Work out the finished part from the listing and answer in its coordinate system (mm). A direction names the side the tool comes from. Coordinates: 2 decimals unless noted, no trailing zeros. Write each loop counter-clockwise with the first axis right and the second up, starting at its lowest first coordinate (ties: lowest second). Pieces come first, ordered by that corner, then holes. Notation, with made-up numbers: (65, 33.5) - (116, 33.5) arc R32 cw to (116, 64.5) - close; hole circle Ø7 at (54, -36.75). An arc over 180 degrees is marked (long way). One line per item, written item: value.
```python
from build123d import *

# Parameters (mm, degrees)
SKETCH1_R               = 15.875
BOSS_EXTRUDE1_DEPTH     = 4.318
SKETCH4_R               = 9.398
BOSS_EXTRUDE2_DEPTH     = 12.954
SKETCH5_R               = 2.921
CUT_EXTRUDE1_DEPTH      = 26.919825732
CUT_EXTRUDE1_DEPTH_BACK = 3.302
SKETCH6_R               = 1.4605
SKETCH6_R_2             = 1.73706236
CUT_EXTRUDE2_DEPTH      = 26.919825732
CUT_EXTRUDE2_DEPTH_BACK = 26.919825732
SKETCH10_R              = 1.27
CUT_EXTRUDE6_DEPTH      = 29.325840394
SKETCH12_R              = 9.398
SKETCH12_R_2            = 8.4455
CUT_EXTRUDE8_DEPTH      = 11.684
CUT_EXTRUDE9_DEPTH      = 10.16


with BuildPart() as part:
    # Sketch1 → Boss-Extrude1 (new body)
    with BuildSketch(Plane(origin=(0, 0, 0), x_dir=(1, 0, 0), z_dir=(0, 1, 0))):
        with Locations(Location((0, 0, 0), (0, 0, 270))):
            Circle(SKETCH1_R)
    extrude(amount=BOSS_EXTRUDE1_DEPTH)

    # Sketch4 → Boss-Extrude2 (add)
    with BuildSketch(Plane(origin=(0, 4.318, 0), x_dir=(1, 0, 0), z_dir=(0, 1, 0))):
        with Locations(Location((0, 0, 0), (0, 0, 270))):
            Circle(SKETCH4_R)
    extrude(amount=BOSS_EXTRUDE2_DEPTH)

    # Sketch5 → Cut-Extrude1 (cut, two sides)
    with BuildSketch(Plane(origin=(0, 4.318, 0), x_dir=(1, 0, 0), z_dir=(0, 1, 0))) as cut_extrude1_sk:
        with Locations(Location((-11.43, 0, 0), (0, 0, 40.395058429))):
            Circle(SKETCH5_R)
        with Locations(Location((11.43, 0, 0), (0, 0, 139.604941571))):
            Circle(SKETCH5_R)
    extrude(amount=CUT_EXTRUDE1_DEPTH, mode=Mode.SUBTRACT)
    extrude(cut_extrude1_sk.sketch, amount=-CUT_EXTRUDE1_DEPTH_BACK, mode=Mode.SUBTRACT)

    # Sketch6 → Cut-Extrude2 (cut, two sides)
    with BuildSketch(Plane(origin=(0, 4.318, 0), x_dir=(1, 0, 0), z_dir=(0, 1, 0))) as cut_extrude2_sk:
        with Locations(Location((-11.43, 0, 0), (0, 0, 270))):
            Circle(SKETCH6_R)
        with Locations(Location((11.43, 0, 0), (0, 0, 270))):
            Circle(SKETCH6_R_2)
    extrude(amount=CUT_EXTRUDE2_DEPTH, mode=Mode.SUBTRACT)
    extrude(cut_extrude2_sk.sketch, amount=-CUT_EXTRUDE2_DEPTH_BACK, mode=Mode.SUBTRACT)

    # Sketch10 → Cut-Extrude6 (cut, through all)
    with BuildSketch(Plane(origin=(0, 17.272, 0), x_dir=(1, 0, 0), z_dir=(0, 1, 0))):
        with Locations(Location((0, 5.08, 0), (0, 0, 270))):
            Circle(SKETCH10_R)
        with Locations(Location((0, -5.08, 0), (0, 0, 270))):
            Circle(SKETCH10_R)
        with Locations(Location((5.08, 0, 0), (0, 0, 270))):
            Circle(SKETCH10_R)
        with Locations(Location((-5.08, 0, 0), (0, 0, 270))):
            Circle(SKETCH10_R)
    extrude(amount=-CUT_EXTRUDE6_DEPTH, mode=Mode.SUBTRACT)

    # Sketch12 → Cut-Extrude8 (cut)
    with BuildSketch(Plane(origin=(0, 17.272, 0), x_dir=(1, 0, 0), z_dir=(0, 1, 0))):
        Circle(SKETCH12_R)
        with Locations(Location((0, 0, 0), (0, 0, 270))):
            Circle(SKETCH12_R_2, mode=Mode.SUBTRACT)
    extrude(amount=-CUT_EXTRUDE8_DEPTH, mode=Mode.SUBTRACT)

    # Sketch13 → Cut-Extrude9 (cut)
    with BuildSketch(Plane.XZ):
        Polygon((7.426351494, 0), (6.253175747, 2.032), (3.906824253, 2.032), (2.733648506, 0), (3.906824253, -2.032), (6.253175747, -2.032), align=None)
        Polygon((2.346351494, -5.08), (1.173175747, -3.048), (-1.173175747, -3.048), (-2.346351494, -5.08), (-1.173175747, -7.112), (1.173175747, -7.112), align=None)
        Polygon((-2.733648506, 0), (-3.906824253, 2.032), (-6.253175747, 2.032), (-7.426351494, 0), (-6.253175747, -2.032), (-3.906824253, -2.032), align=None)
        Polygon((2.346351494, 5.08), (1.173175747, 7.112), (-1.173175747, 7.112), (-2.346351494, 5.08), (-1.173175747, 3.048), (1.173175747, 3.048), align=None)
    extrude(amount=-CUT_EXTRUDE9_DEPTH, mode=Mode.SUBTRACT)


solid = part.part
```
Item 1: Given pin 1 (1.2 mm diameter, centred on x = 0.5, z = 5, fed in from -Y); pin 2 (6 mm diameter, centred on x = -12.5, y = 3, fed in from -Z); pin 3 (8 mm diameter, centred on x = 8.5, y = 12.5, fed in from -Z); pin 4 (0.7 mm diameter, centred on x = -5.5, y = 7, fed in from +Z), each flat-ended and moving along its own axis, determine where each tip first touches the part or whether it passes through.
Evaluation:
pin 1: passes through
pin 2: stops at z = -12.72
pin 3: stops at z = -7.15
pin 4: stops at z = 6.69
Item 2: Determine the mould class of faces 4 (the face through (-0.18, 4.944, 9.396)), 5 (the face through (1.75, 5.01, -6.11)), 6 (the face through (0, 17.272, 0)) for opening direction X: +X half, -X half, draft (parallel to the pull), parting line (faces both ways), or undercut.
Evaluation:
face 4: parting line
face 5: undercut
face 6: draft
Item 3: Section A-A, the plane x = 0 is taken. Give the number of separate pieces and of enclosed holes in the cut face, then the cut area to 3 significant figures.
Evaluation:
separate pieces: 3
enclosed holes: 0
area: 240 mm2
Item 4: Which of the six approach directions +Z, -Z, +X, -X, +Y, -Y give full straight-line access (tool end or side, diameter ignored) to faces 1 (the face through (-1.77, 5.01, -6.08)), 2 (the face through (2.537, 11.512, 8.056)), 3 (the face through (-12.856, 0.515, -0.317))?
Evaluation:
face 1: -Y
face 2: +Y
face 3: +Y, -Y
Item 5: Section B-B, the plane y = 3.5 is taken. Determine the outline of the cut face in (x, z) (3 decimals).
Evaluation:
outline: circle Ø31.75 at (0, 0); hole circle Ø5.842 at (-11.43, 0); hole (-7.426, 0) - (-6.253, -2.032) - (-3.907, -2.032) - (-2.734, 0) - (-3.907, 2.032) - (-6.253, 2.032) - close; hole (-2.346, -5.08) - (-1.173, -7.112) - (1.173, -7.112) - (2.346, -5.08) - (1.173, -3.048) - (-1.173, -3.048) - close; hole (-2.346, 5.08) - (-1.173, 3.048) - (1.173, 3.048) - (2.346, 5.08) - (1.173, 7.112) - (-1.173, 7.112) - close; hole (2.734, 0) - (3.907, -2.032) - (6.253, -2.032) - (7.426, 0) - (6.253, 2.032) - (3.907, 2.032) - close; hole circle Ø5.842 at (11.43, 0)
Item 6: Section D-D, the plane x = 5.08 is taken. Determine the outline of the cut face in (y, z), then the cut area to 3 significant figures.
Evaluation:
outline: (0, -15.04) - (4.32, -15.04) - (4.32, -7.91) - (5.59, -7.91) - (5.59, -6.75) - (17.27, -6.75) - (17.27, -1.27) - (10.16, -1.27) - (10.16, -2.03) - (0, -2.03) - close; (0, 2.03) - (10.16, 2.03) - (10.16, 1.27) - (17.27, 1.27) - (17.27, 6.75) - (5.59, 6.75) - (5.59, 7.91) - (4.32, 7.91) - (4.32, 15.04) - (0, 15.04) - close
area: 248 mm2
Item 7: Consider probe 1 along X at (y, z) = (2, 0) (3 decimals); probe 2 along X at (y, z) = (14.75, 0); probe 3 along Y at (x, z) = (4.5, 13.5). Determine where each line is inside the solid, lowest interval first.
Evaluation:
probe 1: x = -15.875 to -14.351, -8.509 to -7.426, -2.734 to 2.734, 7.426 to 8.509, 14.351 to 15.875
probe 2: x = -8.45 to -6.35, -3.81 to 3.81, 6.35 to 8.45
probe 3: y = 0 to 4.32
Item 8: Section C-C, the plane y = 6 is taken. Determine the outline of the cut face in (x, z), then the cut area to 3 significant figures.
Evaluation:
outline: circle Ø16.89 at (0, 0); hole (-7.43, 0) - (-6.25, -2.03) - (-3.91, -2.03) - (-2.73, 0) - (-3.91, 2.03) - (-6.25, 2.03) - close; hole (-2.35, -5.08) - (-1.17, -7.11) - (1.17, -7.11) - (2.35, -5.08) - (1.17, -3.05) - (-1.17, -3.05) - close; hole (-2.35, 5.08) - (-1.17, 3.05) - (1.17, 3.05) - (2.35, 5.08) - (1.17, 7.11) - (-1.17, 7.11) - close; hole (2.73, 0) - (3.91, -2.03) - (6.25, -2.03) - (7.43, 0) - (6.25, 2.03) - (3.91, 2.03) - close
area: 167 mm2
